Here's how the part is built. I have some questions about the finished solid (model axes, mm). Give positions to 0.01 mm unless a question says otherwise; leave off trailing zeros. Loops run counter-clockwise (first coordinate to the right, second up) from the corner with the lowest first, then second, coordinate; pieces in that order, holes last. Notation, with made-up numbers: (88, 87.5) - (123, 87.5) arc R22 cw to (123, 98.5) - close; hole circle Ø9 at (37.25, 85.5). An arc over 180 degrees is marked (long way). Use a Markdown table: item, result.
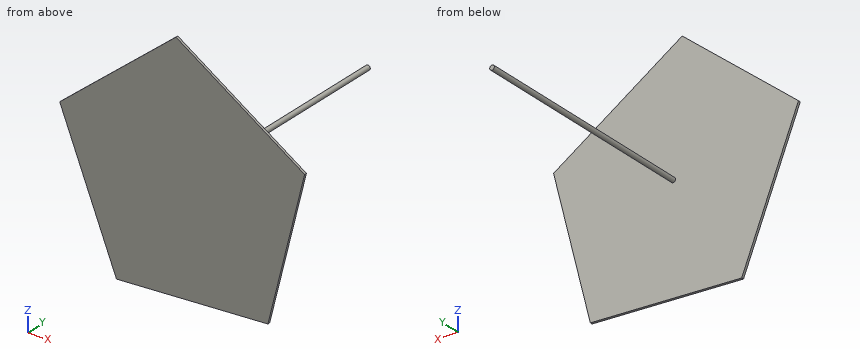
from build123d import *

# Parameters (mm, degrees)
BOSS_EXTRUDE3_DEPTH = 2.54
SKETCH4_R           = 2.54
BOSS_EXTRUDE4_DEPTH = 254


with BuildPart() as part:
    # Sketch3 → Boss-Extrude3 (new body)
    with BuildSketch(Plane(origin=(0, 0, 0), x_dir=(1, 0, 0), z_dir=(0, 1, 0))):
        Polygon((90.212065812, 107.592372069), (-74.449365126, 119.044644473), (-136.224303901, -34.018735606), (-9.741884778, -140.069379332), (130.203487993, -52.548901604), align=None)
    extrude(amount=BOSS_EXTRUDE3_DEPTH)

    # Sketch4 → Boss-Extrude4 (add)
    with BuildSketch(Plane(origin=(0, 2.54, 0), x_dir=(1, 0, 0), z_dir=(0, 1, 0))):
        with Locations(Location((0, -2.079529354, 0), (0, 0, 270))):
            Circle(SKETCH4_R)
    extrude(amount=BOSS_EXTRUDE4_DEPTH)


solid = part.part
(1) Suppose I cut it at A-A on y = 37.5. Write out the boundary of the cut face in (x, z), plus the area to 3 significant figures.
A:
| item | result |
|---|---|
| outline | circle Ø5.08 at (0, 2.08) |
| area | 20.3 mm2 |
(2) Will these pins go through, and if not, where does the flat tip stop? pin 1 (8 mm diameter, centred on x = -88.5, z = 67, fed in from +Y); pin 2 (2 mm diameter, centred on x = 2, z = -55.5, fed in from -Y).
A:
| item | result |
|---|---|
| pin 1 | y = 2.54 |
| pin 2 | y = 0 |
(3) Suppose I cut it at B-B on x = 81. Write out the boundary of the cut face in (y, z).
A:
| item | result |
|---|---|
| outline | (0, -108.23) - (2.54, -108.23) - (2.54, 83.32) - (0, 83.32) - close |
(4) Suppose I cut it at C-C on z = 81.5. Write out the boundary of the cut face in (x, y), plus the area to 3 significant figures.
A:
| item | result |
|---|---|
| outline | (-79.6, 0) - (83.91, 0) - (83.91, 2.54) - (-79.6, 2.54) - close |
| area | 415 mm2 |
(5) If I drill on line 1 (Y direction, x = -17.5, z = 63.5), over which ranges is the centre line in solid material (lowest first)?
A:
| item | result |
|---|---|
| line 1 | 0 to 2.54 |
